Here's the drawing with two shaded views (mm, measured from the low corner). I have some questions. A direction names the side the tool comes from. Coordinates: 2 decimals unless noted, no trailing zeros. Order: outer loops, then holes, each group sorted by start corner. A loop starts at its lowest first (then second) coordinate and runs counter-clockwise, first axis right, second up. Notation, with made-up numbers: (86.25, 68) -> (116.25, 68) arc R16 cw to (116.25, 94) -> close; hole circle Ø6 at (43.25, 37.25). An arc over 180 degrees is marked (long way). Answer as a JSON object with one key per item and string values. Group by question number.
(1) I want a section at A-A, the plane z = 6. List the corners of the cut face in (x, y) for me, plus the area to 3 significant figures.
(2) I want a section at B-B, the plane x = 10.3. List the corners of the cut face in (y, z) for me.
(3) I want a section at D-D, the plane x = 40. List the corners of the cut face in (y, z) for me, plus the area to 3 significant figures.
(4) If we mould it in two halves opening along Z, with no side actions, what happens to the marked faces 3, 4 and 5? For each: pulls with the +Z half, pulls with the -Z half, needs draft (parallel to the pull), parting line crosses it, or undercut.
(5) For pin 1 (3 mm diameter, centred on y = 17.5, z = 6.5, fed in from -X); pin 2 (1 mm diameter, centred on x = 23, y = 13, fed in from +Z); pin 3 (0.5 mm diameter, centred on y = 12.5, z = 28.5, fed in from -X), each with a flat end and sliding along its axis, tell me the tip position at first contact or that it passes through.
(6) Which directions (+Z, -Z, +X, -X, +Y, -Y) give clear straight access to the entire face, cutting with the end or side of a thin tool? Please do the marked faces 1 and 2.
(7) I want a section at C-C, the plane y = 9.8. List the corners of the cut face in (x, z) for me.
(8) I need wall thicknesses on line 1 (Y direction, x = 45, z = 28); line 2 (Y direction, x = 10.3, z = 0.7); line 3 (Z direction, x = 43.5, y = 10.75). Which ranges of each line are inside material? Lowest first, please.
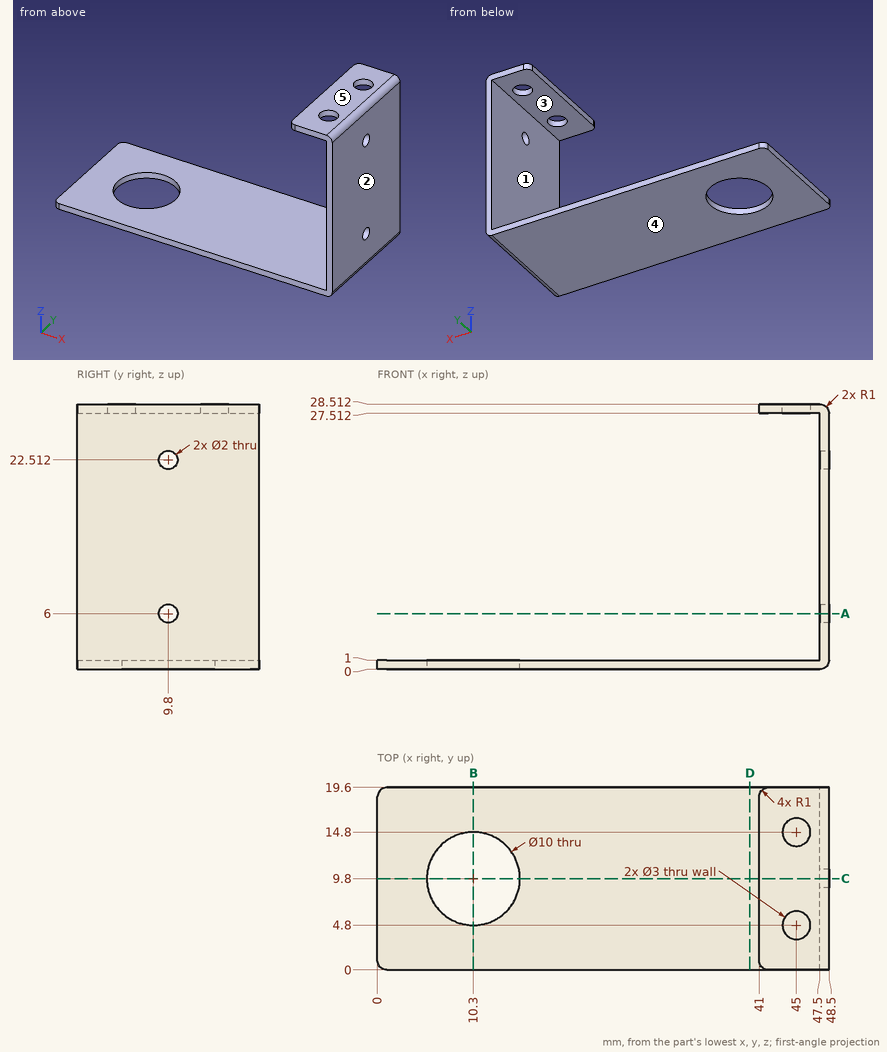
Computed values:
{
 "1": {"outline": "(47.5, 0) -> (48.5, 0) -> (48.5, 8.8) -> (47.5, 8.8) -> close; (47.5, 10.8) -> (48.5, 10.8) -> (48.5, 19.6) -> (47.5, 19.6) -> close", "area": "17.6 mm2"},
 "2": {"outline": "(0, 0) -> (4.8, 0) -> (4.8, 1) -> (0, 1) -> close; (14.8, 0) -> (19.6, 0) -> (19.6, 1) -> (14.8, 1) -> close"},
 "3": {"outline": "(0, 0) -> (19.6, 0) -> (19.6, 1) -> (0, 1) -> close", "area": "19.6 mm2"},
 "4": {"face 3": "undercut", "face 4": "pulls with the -Z half", "face 5": "pulls with the +Z half"},
 "5": {"pin 1": "stops at x = 47.5", "pin 2": "stops at z = 1", "pin 3": "stops at x = 41"},
 "6": {"face 1": "-X, +Y, -Y", "face 2": "+Z, -Z, +X, +Y, -Y"},
 "7": {"outline": "(0, 0) -> (5.3, 0) -> (5.3, 1) -> (0, 1) -> close; (15.3, 0) -> (47.5, 0) arc R1 ccw to (48.5, 1) -> (48.5, 5) -> (47.5, 5) -> (47.5, 1) -> (15.3, 1) -> close; (41, 27.51) -> (47.5, 27.51) -> (47.5, 23.51) -> (48.5, 23.51) -> (48.5, 27.51) arc R1 ccw to (47.5, 28.51) -> (41, 28.51) -> close; (47.5, 7) -> (48.5, 7) -> (48.5, 21.51) -> (47.5, 21.51) -> close"},
 "8": {"line 1": "y = 0 to 3.3, 6.3 to 13.3, 16.3 to 19.6", "line 2": "y = 0 to 4.8, 14.8 to 19.6", "line 3": "z = 0 to 1, 27.51 to 28.51"}
}
